Check sheet for the modelled part. Datum: model origin and axes. Units: mm. Give positions to 0.01 mm unless a question says otherwise; leave off trailing zeros. Loops run counter-clockwise (first coordinate to the right, second up) from the corner with the lowest first, then second, coordinate; pieces in that order, holes last. Notation, with made-up numbers: M -1.5,19.25 L 4.5,19.25 A36 cw 4.5,53.25 Z; hole C 88,76.5 d8. An arc over 180 degrees is marked long. Put each result on its own line as item: value. Start each with the question number.
```python
from build123d import *

# Parameters (mm, degrees)
SKETCH1_R                             = 6.35
BOSS_EXTRUDE1_DEPTH                   = 11.90625
F_1_4_20_TAPPED_HOLE1_D               = 5.1054
F_1_4_20_TAPPED_HOLE1_DEPTH           = 16.51
F_1_4_20_TAPPED_HOLE1_TIP             = 1.533816902
F_1_4_20_TAPPED_HOLE1_ON_FACE_2_D     = 5.1054
F_1_4_20_TAPPED_HOLE1_ON_FACE_2_DEPTH = 16.51
F_1_4_20_TAPPED_HOLE1_ON_FACE_2_TIP   = 1.533816902


with BuildPart() as part:
    # Sketch1 → Boss-Extrude1 (new, symmetric)
    with BuildSketch(Plane.XY):
        Circle(SKETCH1_R)
    extrude(amount=BOSS_EXTRUDE1_DEPTH, both=True)

    # 1/4-20 Tapped Hole1
    with Locations(Plane.XY.offset(11.90625)):
        with Locations((0, 0)):
            Hole(F_1_4_20_TAPPED_HOLE1_D / 2, depth=F_1_4_20_TAPPED_HOLE1_DEPTH)
            with Locations((0, 0, -(F_1_4_20_TAPPED_HOLE1_DEPTH + F_1_4_20_TAPPED_HOLE1_TIP / 2))):  # 118° drill point
                Cone(0, F_1_4_20_TAPPED_HOLE1_D / 2, F_1_4_20_TAPPED_HOLE1_TIP, mode=Mode.SUBTRACT)

    # 1/4-20 Tapped Hole1 on face 2
    with Locations(Plane(origin=(0, 0, -11.90625), x_dir=(-1, 0, 0), z_dir=(0, 0, -1))):
        with Locations((0, 0)):
            Hole(F_1_4_20_TAPPED_HOLE1_ON_FACE_2_D / 2, depth=F_1_4_20_TAPPED_HOLE1_ON_FACE_2_DEPTH)
            with Locations((0, 0, -(F_1_4_20_TAPPED_HOLE1_ON_FACE_2_DEPTH + F_1_4_20_TAPPED_HOLE1_ON_FACE_2_TIP / 2))):  # 118° drill point
                Cone(0, F_1_4_20_TAPPED_HOLE1_ON_FACE_2_D / 2, F_1_4_20_TAPPED_HOLE1_ON_FACE_2_TIP, mode=Mode.SUBTRACT)


solid = part.part
```
Q1. Section check C-C, the plane z = 9.5. Record the cut outline in (x, y).
Q2. Section check B-B, the plane y = -0.5. Record the cut outline in (x, z).
Q3. Section check A-A, the plane x = 0. Record the cut outline in (y, z).
Q4. Depth check by flat-ended pin: P1, Ø2, axis at y = -4, z = -7.5, coming from the +X side; P2, Ø3, axis at x = 0, y = 0, coming from the +Z side. Enter the tip coordinate at first touch or a pass-through.
Q5. Section check D-D, the plane x = 4. Record the cut outline in (y, z).
Q6. Thickness scan on line 1 along Y through (x, z) = (0, 6.75); line 2 along Y through (x, z) = (-1.25, -5.5); line 3 along X through (y, z) = (-1, -1). Record the ranges inside material, lowest first. Write a range as [from, to].
Found:
1. outline: C 0,0 d12.7; hole C 0,0 d5.11
2. outline: M -6.33,-11.91 L -2.5,-11.91 L -2.5,11.91 L -6.33,11.91 Z; M 2.5,-11.91 L 6.33,-11.91 L 6.33,11.91 L 2.5,11.91 Z
3. outline: M -6.35,-11.91 L -2.55,-11.91 L -2.55,11.91 L -6.35,11.91 Z; M 2.55,-11.91 L 6.35,-11.91 L 6.35,11.91 L 2.55,11.91 Z
4. P1: stops at x = 5.6
4. P2: passes through
5. outline: M -4.93,-11.91 L 4.93,-11.91 L 4.93,11.91 L -4.93,11.91 Z
6. line 1: y = [-6.35, -2.55], [2.55, 6.35]
6. line 2: y = [-6.23, -2.23], [2.23, 6.23]
6. line 3: x = [-6.27, -2.35], [2.35, 6.27]
